Design review of the part built by this model. Coordinates are the model's own, in mm. A direction names the side the tool comes from. Give positions to 0.01 mm unless a question says otherwise; leave off trailing zeros. Write each loop counter-clockwise with the first axis right and the second up, starting at its lowest first coordinate (ties: lowest second). Pieces come first, ordered by that corner, then holes. Notation, with made-up numbers: (-28, -10.5) -> (-2, -10.5) arc R8 ccw to (-2, -2.5) -> close; hole circle Ø11 at (64, -19.75). An arc over 180 degrees is marked (long way). Answer as a JSON object with one key per item and string values.
```python
from build123d import *

# Parameters (mm, degrees)
SKETCH2_R           = 49.53
BOSS_EXTRUDE1_DEPTH = 3.81
SKETCH3_R           = 47.752
BOSS_EXTRUDE2_DEPTH = 3.81
SKETCH5_R           = 3.175
SKETCH5_R_2         = 1.5875
SKETCH5_R_3         = 2.38125
CUT_EXTRUDE1_DEPTH  = 17.526


with BuildPart() as part:
    # Sketch2 → Boss-Extrude1 (new body)
    with BuildSketch(Plane(origin=(0, 0, 0), x_dir=(1, 0, 0), z_dir=(0, 1, 0))):
        with Locations(Location((0, 0, 0), (0, 0, 90))):
            Circle(SKETCH2_R)
    extrude(amount=BOSS_EXTRUDE1_DEPTH)

    # Sketch3 → Boss-Extrude2 (add)
    with BuildSketch(Plane(origin=(0, 3.81, 0), x_dir=(1, 0, 0), z_dir=(0, 1, 0))):
        with Locations(Location((0, 0, 0), (0, 0, 90))):
            Circle(SKETCH3_R)
    extrude(amount=BOSS_EXTRUDE2_DEPTH)

    # Sketch5 → Cut-Extrude1 (cut)
    with BuildSketch(Plane.XZ):
        with Locations(Location((37.1475, 0, 0), (0, 0, 270))):
            Circle(SKETCH5_R)
        with Locations(Location((-37.1475, 0, 0), (0, 0, 270))):
            Circle(SKETCH5_R)
        with Locations(Location((0, 37.1475, 0), (0, 0, 270))):
            Circle(SKETCH5_R_2)
        with Locations(Location((0, 0, 0), (0, 0, 270))):
            Circle(SKETCH5_R_3)
    extrude(amount=-CUT_EXTRUDE1_DEPTH, mode=Mode.SUBTRACT)


solid = part.part
```
(1) We need section B-B, the plane x = 0. State the section outline as (y, z) points (3 decimals).
Here are the results:
{"outline": "(0, -49.53) -> (3.81, -49.53) -> (3.81, -47.752) -> (7.62, -47.752) -> (7.62, -2.381) -> (0, -2.381) -> close; (0, 2.381) -> (7.62, 2.381) -> (7.62, 35.56) -> (0, 35.56) -> close; (0, 38.735) -> (7.62, 38.735) -> (7.62, 47.752) -> (3.81, 47.752) -> (3.81, 49.53) -> (0, 49.53) -> close"}
(2) The part is to be moulded in two halves that separate along Z. For faces 3 (the flat face through (-41, 3.81, 26)), 4 (the cylindrical face through (-14.88, 1.88, -47.24)), 5 (the cylindrical face through (0.477, 3.757, 35.633)), say which applies: +Z half, -Z half, draft (parallel to the pull), parting line (faces both ways), or undercut.
Here are the results:
{"face 3": "draft", "face 4": "parting line", "face 5": "undercut"}
(3) For faces 1 (the cylindrical face through (-14.34, 5.69, -45.55)), 2 (the flat face through (-1, 0, -10)), list the 3-axis set-ups (+Z, -Z, +X, -X, +Y, -Y) from which the entire face can be reached by the end or side of a thin tool; tool diameter is ignored.
Here are the results:
{"face 1": "+Y", "face 2": "+Z, -Z, +X, -X, -Y"}
(4) Clearance check with flat-ended pins moving along their axes: pin 1 (1.5 mm diameter, centred on y = 2.5, z = 11, fed in from -X); pin 2 (1 mm diameter, centred on y = 5, z = 36, fed in from -X); pin 3 (4 mm diameter, centred on y = 6, z = -16.5, fed in from +X). State where each tip first meets the part, or that it passes through.
Here are the results:
{"pin 1": "stops at x = -48.46", "pin 2": "stops at x = -31.94", "pin 3": "stops at x = 45.5"}
(5) We need section A-A, the plane z = 0. State the section outline as (x, y) points.
Here are the results:
{"outline": "(-49.53, 0) -> (-40.32, 0) -> (-40.32, 7.62) -> (-47.75, 7.62) -> (-47.75, 3.81) -> (-49.53, 3.81) -> close; (-33.97, 0) -> (-2.38, 0) -> (-2.38, 7.62) -> (-33.97, 7.62) -> close; (2.38, 0) -> (33.97, 0) -> (33.97, 7.62) -> (2.38, 7.62) -> close; (40.32, 0) -> (49.53, 0) -> (49.53, 3.81) -> (47.75, 3.81) -> (47.75, 7.62) -> (40.32, 7.62) -> close"}
(6) We need section C-C, the plane y = 1.75. Give the number of separate pieces and of enclosed holes in the cut face, then the cut area to 3 significant figures.
Here are the results:
{"separate pieces": "1", "enclosed holes": "4", "area": "7,620 mm²"}
(7) We need section D-D, the plane z = -37. State the section outline as (x, y) points.
Here are the results:
{"outline": "(-32.93, 0) -> (32.93, 0) -> (32.93, 3.81) -> (30.19, 3.81) -> (30.19, 7.62) -> (-30.19, 7.62) -> (-30.19, 3.81) -> (-32.93, 3.81) -> close"}
(8) For line 1 along X through (y, z) = (5.75, 0); line 2 along X through (y, z) = (2.25, 0); line 3 along Z through (x, y) = (1, 3.25), list the stretches that pass through material, from the lowest coordinate up.
Here are the results:
{"line 1": "x = -47.75 to -40.32, -33.97 to -2.38, 2.38 to 33.97, 40.32 to 47.75", "line 2": "x = -49.53 to -40.32, -33.97 to -2.38, 2.38 to 33.97, 40.32 to 49.53", "line 3": "z = -49.52 to -2.16, 2.16 to 35.91, 38.38 to 49.52"}
